Check sheet for the drawn part. Datum: minimum x, y, z corner. Units: mm. A direction names the side the tool comes from. Round coordinates to 2 decimals unless told otherwise and drop trailing zeros. Write each loop counter-clockwise with the first axis right and the second up, starting at its lowest first coordinate (ties: lowest second). Pieces come first, ordered by that corner, then holes. Notation, with made-up numbers: M -31,13.5 L 15,13.5 A14 cw 15,26.5 Z; hole C 14,84 d5. An arc over 180 degrees is marked long. One line per item, written item: value. Start each with the question number.
1. Section check C-C (y = 32.5). Record the boundary of the cut face in (x, z), and give its area (3 significant figures).
2. Section check D-D (z = 82.5). Record the boundary of the cut face in (x, y).
3. Release check for a two-part mould opening along Y. For the marked faces 3, 4 and 5 record: pulls with the +Y half, pulls with the -Y half, needs draft (parallel to the pull), parting line crosses it, or undercut.
4. Depth check by flat-ended pin: P1, Ø7.5, axis at x = 10.5, z = 15.5, coming from the -Y side; P2, Ø2.5, axis at x = 12, z = 18.5, coming from the +Y side; P3, Ø4, axis at x = 2, y = 32, coming from the -Z side; P4, Ø15.5, axis at y = 53.5, z = 10.5, coming from the -X side. Enter the tip coordinate at first touch or a pass-through.
5. Scan lines: probe 1 along Y at (x, z) = (8.75, 16.5); probe 2 along Z at (x, y) = (11.5, 49); probe 3 along Z at (x, y) = (11, 36.5). Record each from-to range of solid material in increasing order. Write a range as [from, to].
6. Section check A-A (y = 44.45). Record the boundary of the cut face in (x, z) (1 decimal).
7. Access from +Z, -Z, +X, -X, +Y, -Y to the whole of each face (thin tool, end or side, straight path). Record for the marked faces 1 and 2.
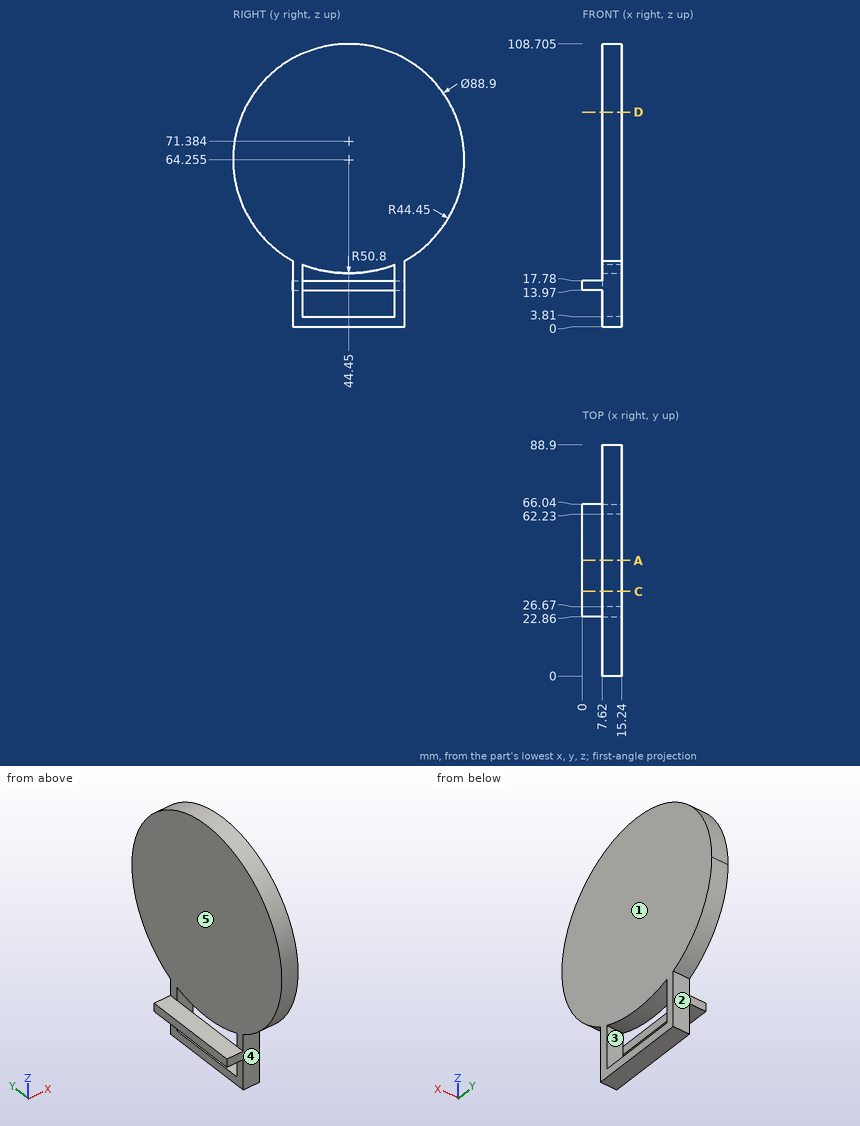
Result sheet:
1. outline: M 0,13.97 L 7.62,13.97 L 7.62,17.78 L 0,17.78 Z; M 7.62,0 L 15.24,0 L 15.24,3.81 L 7.62,3.81 Z; M 7.62,22.01 L 15.24,22.01 L 15.24,107.07 L 7.62,107.07 Z
1. area: 706 mm2
2. outline: M 7.62,3.92 L 15.24,3.92 L 15.24,84.98 L 7.62,84.98 Z
3. face 3: undercut
3. face 4: pulls with the -Y half
3. face 5: needs draft
4. P1: stops at y = 22.86
4. P2: stops at y = 66.04
4. P3: stops at z = 13.97
4. P4: stops at x = 0
5. probe 1: y = [22.86, 26.67], [62.23, 66.04]
5. probe 2: z = [0, 3.81], [20.79, 108.47]
5. probe 3: z = [0, 3.81], [21.21, 107.99]
6. outline: M 0,14 L 7.6,14 L 7.6,17.8 L 0,17.8 Z; M 7.6,0 L 15.2,0 L 15.2,3.8 L 7.6,3.8 Z; M 7.6,20.6 L 15.2,20.6 L 15.2,108.7 L 7.6,108.7 Z
7. face 1: +Z, -Z, +X, +Y, -Y
7. face 2: -Z, +X, -X, +Y
